```python
from build123d import *

# Parameters (mm, degrees)
EXTRUDE_1_DEPTH     = 10
SKETCH_2_R          = 1.5
CUT_EXTRUDE_1_DEPTH = 6
SKETCH_3_R          = 1.5
CUT_EXTRUDE_2_DEPTH = 5
SKETCH_4_R          = 1.5
CUT_EXTRUDE_3_DEPTH = 10
SKETCH_5_R          = 1.5
CUT_EXTRUDE_4_DEPTH = 10
SKETCH_6_R          = 1.5
CUT_EXTRUDE_5_DEPTH = 10


with BuildPart() as part:
    # 草图1 → 凸台-拉伸1 (new body)
    with BuildSketch(Plane(origin=(0, 0, 0), x_dir=(0, 0, -1), z_dir=(1, 0, 0))):
        Polygon((96, 112.5), (200, 112.5), (200, -112.5), (-200, -112.5), (-200, 112.5), (-96, 112.5), (-96, 82.5), (-85, 82.5), (-85, 112.5), (85, 112.5), (85, 82.5), (96, 82.5), align=None)
    extrude(amount=EXTRUDE_1_DEPTH)

    # 草图2 → 切除-拉伸1 (cut)
    with BuildSketch(Plane.ZY):
        with Locations((-84, -105.5)):
            Circle(SKETCH_2_R)
        with Locations((-66, -105.5)):
            Circle(SKETCH_2_R)
        with Locations((-9, -105.5)):
            Circle(SKETCH_2_R)
        with Locations((9, -105.5)):
            Circle(SKETCH_2_R)
        with Locations((66, -105.5)):
            Circle(SKETCH_2_R)
        with Locations((84, -105.5)):
            Circle(SKETCH_2_R)
    extrude(amount=-CUT_EXTRUDE_1_DEPTH, mode=Mode.SUBTRACT)

    # 草图3 → 切除-拉伸2 (cut)
    with BuildSketch(Plane(origin=(10, 0, 0), x_dir=(0, 0, -1), z_dir=(1, 0, 0))):
        with Locations((197, -91.5)):
            Circle(SKETCH_3_R)
        with Locations((191, -91.5)):
            Circle(SKETCH_3_R)
        with Locations((191, 73.5)):
            Circle(SKETCH_3_R)
        with Locations((197, 73.5)):
            Circle(SKETCH_3_R)
    cut_extrude_2 = extrude(amount=-CUT_EXTRUDE_2_DEPTH, mode=Mode.SUBTRACT)

    # 镜向1: 切除-拉伸2 across plane
    add(cut_extrude_2.mirror(Plane.XY), mode=Mode.SUBTRACT)

    # 草图4 → 切除-拉伸3 (cut)
    with BuildSketch(Plane(origin=(10, 0, 0), x_dir=(0, 0, -1), z_dir=(1, 0, 0))):
        with Locations((7.43, -92.5)):
            Circle(SKETCH_4_R)
        with Locations((-7.57, -92.5)):
            Circle(SKETCH_4_R)
    extrude(amount=-CUT_EXTRUDE_3_DEPTH, mode=Mode.SUBTRACT)

    # 草图5 → 切除-拉伸4 (cut)
    with BuildSketch(Plane(origin=(10, 0, 0), x_dir=(0, 0, -1), z_dir=(1, 0, 0))):
        with Locations((-80, 82.5)):
            Circle(SKETCH_5_R)
        with Locations((-65, 82.5)):
            Circle(SKETCH_5_R)
    cut_extrude_4 = extrude(amount=-CUT_EXTRUDE_4_DEPTH, mode=Mode.SUBTRACT)

    # 镜向2: 切除-拉伸4 across plane
    add(cut_extrude_4.mirror(Plane.XY), mode=Mode.SUBTRACT)

    # 草图6 → 切除-拉伸5 (cut)
    with BuildSketch(Plane(origin=(10, 0, 0), x_dir=(0, 0, -1), z_dir=(1, 0, 0))):
        with Locations((-7.5, 22.5)):
            Circle(SKETCH_6_R)
        with Locations((7.5, 22.5)):
            Circle(SKETCH_6_R)
    extrude(amount=-CUT_EXTRUDE_5_DEPTH, mode=Mode.SUBTRACT)


solid = part.part
```
Could you check a few things on this model? Use its own coordinates, in mm. A direction names the side the tool comes from. Round coordinates to 2 decimals unless told otherwise and drop trailing zeros.
Q1. Thinking about a two-plate mould opening in Y: for faces 1 (the flat face through (5, 112.5, -147)), 2 (the flat face through (5, -112.5, -3)), 3 (the flat face through (5, 2, -200)), which applies, pulls with the +Y half, pulls with the -Y half, needs draft (parallel to the pull), parting line crosses it, or undercut?
Q2. For P1, Ø1.5, axis at y = -105, z = -9, coming from the -X side; P2, Ø1.8, axis at y = 82.5, z = -80, coming from the -X side; P3, Ø2.5, axis at y = 73.5, z = -191, coming from the +X side, each with a flat end and sliding along its axis, tell me the tip position at first contact or that it passes through.
Q3. Please list where these lines run through material, in increasing order: L1, parallel to Z at x = 5, y = 95.5; L2, parallel to Z at x = 2.75, y = -92.5; L3, parallel to Z at x = 8.15, y = 73.5.
Q4. On a 3-axis mill with a long thin cutter (end or side, diameter ignored), from which of +Z, -Z, +X, -X, +Y, -Y can I reach the whole of each face in a straight line? I mean faces 4 (the flat face through (5, -2, 200)), 5 (the flat face through (5, 98, 96)). Say none if no direction works.
Answer below:
1. face 1: pulls with the +Y half
1. face 2: pulls with the -Y half
1. face 3: needs draft
2. P1: stops at x = 6
2. P2: passes through
2. P3: stops at x = 5
3. L1: z = -200 to -96, -85 to 85, 96 to 200
3. L2: z = -200 to -8.93, -5.93 to 6.07, 9.07 to 200
3. L3: z = -200 to -198.5, -195.5 to -192.5, -189.5 to 189.5, 192.5 to 195.5, 198.5 to 200
4. face 4: +Z, +X, -X, +Y, -Y
4. face 5: +X, -X, +Y
